The listing builds one solid part. Answer for the finished solid, in the listing's coordinates (mm). A direction names the side the tool comes from. Coordinates: 2 decimals unless noted, no trailing zeros. Order: outer loops, then holes, each group sorted by start corner. A loop starts at its lowest first (then second) coordinate and runs counter-clockwise, first axis right, second up.
from build123d import *

# Parameters (mm, degrees)
BOSS_EXTRU_1_DEPTH           = 10.7
ESQUISSE2_R                  = 1.35
ENL_V_MAT_EXTRU_1_DEPTH      = 1
ENL_V_MAT_EXTRU_1_DEPTH_BACK = 11.7
CONG_1_R                     = 1


with BuildPart() as part:
    # Esquisse1 → Boss.-Extru.1 (new body)
    with BuildSketch(Plane.XY):
        Polygon((-12.5, 0), (12.5, 0), (12.5, 24), (17.5, 24), (17.5, -5), (-17.5, -5), (-17.5, 24), (-12.5, 24), align=None)
    extrude(amount=BOSS_EXTRU_1_DEPTH)

    # Esquisse2 → Enlèv. mat.-Extru.1 (cut, two sides)
    with BuildSketch(Plane.XY.offset(10.7)) as enl_v_mat_extru_1_sk:
        with Locations((-15, 21)):
            Circle(ESQUISSE2_R)
        with Locations((-15, 4)):
            Circle(ESQUISSE2_R)
        with Locations((15, 4)):
            Circle(ESQUISSE2_R)
        with Locations((15, 21)):
            Circle(ESQUISSE2_R)
    extrude(amount=ENL_V_MAT_EXTRU_1_DEPTH, mode=Mode.SUBTRACT)
    extrude(enl_v_mat_extru_1_sk.sketch, amount=-ENL_V_MAT_EXTRU_1_DEPTH_BACK, mode=Mode.SUBTRACT)

    # Congé1
    cong_1_edges = [part.edges().sort_by_distance(p)[0] for p in [
        (12.5, 24, 5.35),
        (17.5, 24, 5.35),
        (17.5, -5, 5.35),
        (-17.5, -5, 5.35),
        (-17.5, 24, 5.35),
        (-12.5, 24, 5.35),
        (-12.5, 0, 5.35),
        (12.5, 0, 5.35),
    ]]
    fillet(cong_1_edges, radius=CONG_1_R)


solid = part.part
1) A tool of negligible diameter and unlimited length cuts with its end or side. For faces 5 (the face through (13.65, 4.06, 5.42)), 6 (the face through (-12.5, 12, 5)), from which of +Z, -Z, +X, -X, +Y, -Y can it reach the whole face along a straight path? Write none if from no direction.
2) Section C-C (z = 9) is taken. Give the vertices of the cut face in (x, y).
3) Consider L1, parallel to Y at x = -15, z = 5.5; L2, parallel to X at y = 8, z = 7.75; L3, parallel to Y at x = -1, z = 9. Determine where each line is inside the solid, lowest interval first.
4) Section B-B (x = 15) is taken. Give the vertices of the cut face in (y, z).
5) Section A-A (y = 14.5) is taken. Give the vertices of the cut face in (x, z), then the cut area to 3 significant figures.
6) Each of these flat-tipped pins is pushed along its axis until it touches: P1, Ø4, axis at x = -5, z = 8, coming from the +Y side; P2, Ø6, axis at x = -10.5, y = 15.5, coming from the +Z side. Where does it stop, or does it pass through?
7) Determine the mould class of faces 1 (the face through (-16.07, 3.18, 5.42)), 2 (the face through (-17.199, 23.715, 5.425)), 3 (the face through (17.199, 23.715, 5.425)), 4 (the face through (0, -1, 0)) for opening direction X: released by +X, released by -X, zero draft, split by the parting line, or undercut.
8) Section D-D (y = 4.5) is taken. Give the vertices of the cut face in (x, z), then the cut area to 3 significant figures.
Filled sheet:
1. face 5: +Z, -Z
1. face 6: +Z, -Z, +Y
2. outline: (-17.5, -4) arc R1 ccw to (-16.5, -5) - (16.5, -5) arc R1 ccw to (17.5, -4) - (17.5, 23) arc R1 ccw to (16.5, 24) - (13.5, 24) arc R1 ccw to (12.5, 23) - (12.5, 1) arc R1 cw to (11.5, 0) - (-11.5, 0) arc R1 cw to (-12.5, 1) - (-12.5, 23) arc R1 ccw to (-13.5, 24) - (-16.5, 24) arc R1 ccw to (-17.5, 23) - close; hole circle Ø2.7 at (-15, 4); hole circle Ø2.7 at (-15, 21); hole circle Ø2.7 at (15, 4); hole circle Ø2.7 at (15, 21)
3. L1: y = -5 to 2.65, 5.35 to 19.65, 22.35 to 24
3. L2: x = -17.5 to -12.5, 12.5 to 17.5
3. L3: y = -5 to 0
4. outline: (-5, 0) - (2.65, 0) - (2.65, 10.7) - (-5, 10.7) - close; (5.35, 0) - (19.65, 0) - (19.65, 10.7) - (5.35, 10.7) - close; (22.35, 0) - (24, 0) - (24, 10.7) - (22.35, 10.7) - close
5. outline: (-17.5, 0) - (-12.5, 0) - (-12.5, 10.7) - (-17.5, 10.7) - close; (12.5, 0) - (17.5, 0) - (17.5, 10.7) - (12.5, 10.7) - close
5. area: 107 mm2
6. P1: stops at y = 0
6. P2: stops at z = 10.7
7. face 1: undercut
7. face 2: released by -X
7. face 3: released by +X
7. face 4: zero draft
8. outline: (-17.5, 0) - (-16.25, 0) - (-16.25, 10.7) - (-17.5, 10.7) - close; (-13.75, 0) - (-12.5, 0) - (-12.5, 10.7) - (-13.75, 10.7) - close; (12.5, 0) - (13.75, 0) - (13.75, 10.7) - (12.5, 10.7) - close; (16.25, 0) - (17.5, 0) - (17.5, 10.7) - (16.25, 10.7) - close
8. area: 53.3 mm2
